Could you check a few things on this model? Use its own coordinates, in mm. A direction names the side the tool comes from. Coordinates: 2 decimals unless noted, no trailing zeros. Write each loop counter-clockwise with the first axis right and the second up, starting at its lowest first coordinate (ties: lowest second). Pieces come first, ordered by that corner, then holes.
Autodesk Fusion 360 part; units mm, degrees
sketch "Sketch1" plane through (0, 0, 0) normal (0, 0, 1) x (1, 0, 0)
  line L0 (0, 0) -> (7, 0)
  line L1 (7, 0) -> (7, 35)
  line L2 (7, 35) -> (64, 35)
  line L3 (64, 35) -> (64, 0)
  line L4 (64, 0) -> (71, 0)
  line L5 (71, 0) -> (71, 42)
  line L6 (71, 42) -> (0, 42)
  line L7 (0, 42) -> (0, 0)
  dimension "d1" = 7
  dimension "d2" = 35
  dimension "d3" = 57
  dimension "d9" = 7
extrude "Extrude1" add sketch "Sketch1" along normal blind 7
sketch "Sketch2" plane through (0, 0, 7) normal (0, 0, 1) x (-1, 0, 0)
  line L0 (0, -42) -> (0, 0)
  line L1 (0, 0) -> (-7, 0)
  line L2 (-7, 0) -> (-7, -35)
  line L3 (-7, -35) -> (-64, -35)
  line L4 (-64, -35) -> (-64, 0)
  line L5 (-64, 0) -> (-71, 0)
  line L6 (-71, 0) -> (-71, -42)
  line L7 (-71, -42) -> (0, -42)
  line L8 (0, -4) -> (-7, -4)
  line L9 (-64, -4) -> (-71, -4)
  dimension "d10" = 4
extrude "Extrude2" add sketch "Sketch2" along normal blind 7 contours L0 L1 L2 L8 | L4 L5 L6 L9
extrude "Extrude4" add 1 faces at (4.6667, 2.6667, 14) along direction (0, 0, 1) blind 7
extrude "Extrude5" add 1 faces at (66.3333, 2.6667, 14) along direction (0, 0, 1) blind 7
sketch "Sketch5" plane through (0, 42, 0) normal (0, 1, 0) x (-1, 0, 0)
  line L0 (-71, 0) -> (0, 0)
  line L1 (0, 0) -> (0, 7)
  line L2 (0, 7) -> (-71, 7)
  line L3 (-71, 7) -> (-71, 0)
  line L4 (-71, 7) -> (0, 0)
  line L5 (0, 7) -> (-71, 0)
  circle A0 centre (-35.5, 3.5) radius 2
  dimension "d25" = 4
extrude "Extrude7" cut sketch "Sketch5" against normal blind 100 contours L4 L5 A0 | L4 L5 A0 | L4 L5 A0 | L4 L5 A0
sketch "Sketch6" plane through (0, 0, 0) normal (0, -1, 0) x (1, 0, 0)
  line L0 (0, 0) -> (7, 0)
  line L1 (7, 0) -> (7, 21)
  line L2 (7, 21) -> (0, 21)
  line L3 (0, 21) -> (0, 0)
  line L4 (3.5, 21) -> (3.5, 17.5)
  circle A0 centre (3.5, 17.5) radius 1.55
  line L5 (3.5, 17.5) -> (3.5, 10.5)
  circle A1 centre (3.5, 10.5) radius 1.55
  dimension "d28" = 3.5
  dimension "d29" = 3.1
  dimension "d30" = 7
sketch "Sketch7" plane through (0, 0, 0) normal (0, -1, 0) x (1, 0, 0)
  line L0 (64, 0) -> (71, 0)
  line L1 (71, 0) -> (71, 21)
  line L2 (71, 21) -> (64, 21)
  line L3 (64, 21) -> (64, 0)
  line L4 (67.5, 21) -> (67.5, 17.5)
  line L5 (67.5, 17.5) -> (67.5, 10.5)
  circle A0 centre (67.5, 17.5) radius 1.55
  circle A1 centre (67.5, 10.5) radius 1.55
  dimension "d31" = 3.5
  dimension "d32" = 7
  dimension "d33" = 3.1
extrude "Extrude8" cut sketch "Sketch6" sketch "Sketch7" against normal blind 100 contours A1 | L4 A0 L5 | L4 A0 L5 of sketch 2 contours A1 | L4 L5 A0 | L4 L5 A0
extrude "Extrude9" add 2 faces at (6.327, 4, 15.0144) (64.673, 4, 15.0144) along direction (0, 1, 0) blind 2
1. I want a section at C-C on z = 17.5. Please give me the cut outline in (x, y), plus the area to 3 significant figures.
Verdict:
outline: (0, 0) - (1.95, 0) - (1.95, 6) - (0, 6) - close; (5.05, 0) - (7, 0) - (7, 6) - (5.05, 6) - close; (64, 0) - (65.95, 0) - (65.95, 6) - (64, 6) - close; (69.05, 0) - (71, 0) - (71, 6) - (69.05, 6) - close
area: 46.8 mm2
2. Please list where these lines run through material, in increasing order: line 1 along X through (y, z) = (3.3, 10.5); line 2 along X through (y, z) = (4, 11.75); line 3 along Z through (x, y) = (3, 3).
Verdict:
line 1: x = 0 to 1.95, 5.05 to 7, 64 to 65.95, 69.05 to 71
line 2: x = 0 to 2.58, 4.42 to 7, 64 to 66.58, 68.42 to 71
line 3: z = 0 to 9.03, 11.97 to 16.03, 18.97 to 21
3. For pin 1 (10 mm diameter, centred on x = 30, z = 5.5, fed in from -Y); pin 2 (5.5 mm diameter, centred on x = 3.5, z = 10.5, fed in from +Y); pin 3 (3.5 mm diameter, centred on x = 35.5, z = 3.5, fed in from -Y), each with a flat end and sliding along its axis, tell me the tip position at first contact or that it passes through.
Verdict:
pin 1: stops at y = 35
pin 2: stops at y = 6
pin 3: passes through
4. On a 3-axis mill with a long thin cutter (end or side, diameter ignored), from which of +Z, -Z, +X, -X, +Y, -Y can I reach the whole of each face in a straight line? I mean faces 1 (the face through (67, 6, 14)), 2 (the face through (2.27, 2.96, 9.56)), 3 (the face through (64, 14, 6)). Say none if no direction works.
Verdict:
face 1: +Z, +X, -X, +Y
face 2: +Y, -Y
face 3: +Z, -Z, -Y
5. I want a section at D-D on x = 35.5. Please give me the cut outline in (y, z), plus the area to 3 significant figures.
Verdict:
outline: (35, 0) - (42, 0) - (42, 1.5) - (35, 1.5) - close; (35, 5.5) - (42, 5.5) - (42, 7) - (35, 7) - close
area: 21.0 mm2
6. If we mould it in two halves opening along X, with no side actions, what happens to faces 4 (the face through (3, 6, 14)), 5 (the face through (35, 35, 1)), 6 (the face through (68.978, 2.958, 17.966)), 7 (the face through (71, 16, 6))? For each: pulls with the +X half, pulls with the -X half, needs draft (parallel to the pull), parting line crosses it, or undercut.
Verdict:
face 4: needs draft
face 5: undercut
face 6: undercut
face 7: pulls with the +X half
7. I want a section at B-B on y = 39.5. Please give me the cut outline in (x, z), plus the area to 3 significant figures.
Verdict:
outline: (0, 0) - (71, 0) - (71, 7) - (0, 7) - close; hole circle Ø4 at (35.5, 3.5)
area: 484 mm2
8. I want a section at A-A on x = 3.5. Please give me the cut outline in (y, z).
Verdict:
outline: (0, 0) - (42, 0) - (42, 7) - (6, 7) - (6, 8.95) - (0, 8.95) - close; (0, 12.05) - (6, 12.05) - (6, 15.95) - (0, 15.95) - close; (0, 19.05) - (6, 19.05) - (6, 21) - (0, 21) - close
